Read the model definition and answer for the solid it produces. Units are mm, in the model's axes. A direction names the side the tool comes from. Coordinates: 2 decimals unless noted, no trailing zeros. Loops run counter-clockwise (first coordinate to the right, second up) from the corner with the lowest first, then second, coordinate; pieces in that order, holes last. Notation, with made-up numbers: (26, -5) - (82, -5) arc R23 ccw to (82, 25) - close; hole circle Ø6 at (67.5, 66.25). An arc over 180 degrees is marked (long way). One line per question, with ' | ' between items. Start each with the question number.
```python
from build123d import *

# Parameters (mm, degrees)
F0_W     = 42.25
F0_H     = 214
F1_DEPTH = 59
F3_DEPTH = 214
F4_T     = -1.5


with BuildPart() as f1:
    # F0 (on Top) → F1 (new body)
    with BuildSketch(Plane.XY):
        with Locations((21.125, 107)):
            Rectangle(F0_W, F0_H)
    extrude(amount=F1_DEPTH)

    # F2 (on face) → F3 (cut, through all)
    with BuildSketch(Plane(origin=(0, 214, 0), x_dir=(-1, 0, 0), z_dir=(0, 1, 0))):
        Polygon((0, 0), (-42.25, 59), (-42.25, 0), align=None)
    extrude(amount=-F3_DEPTH, mode=Mode.SUBTRACT)

    # F4
    f4_openings = [f1.faces().sort_by_distance(p)[0] for p in [
        (21.125, 107, 29.5),
    ]]
    offset(amount=F4_T, openings=f4_openings)


solid = f1.part
```
1) Given pin 1 Ø2 at (x, y) = (23.5, 86.5) entering from -Z, flat-ended and moving along its own axis, determine where the tip first touches the part or whether it passes through.
2) Find the intervals of material crossed by line 1 along Y through (x, z) = (23, 42); line 2 along X through (y, z) = (43, 35); line 3 along Z through (x, y) = (18, 165.5), in increasing order. Write a range as from..to.
3) The part is cut by section A-A on y = 92. Write down the section's boundary in (x, z), and give its area (3 significant figures).
4) The part is cut by section C-C on x = 39. Write down the section's boundary in (y, z), and give its area (3 significant figures).
5) The part is cut by section B-B on z = 46. Write down the section's boundary in (x, y), and give its area (3 significant figures).
6) Which of the six approach directions +Z, -Z, +X, -X, +Y, -Y give full straight-line access (tool end or side, diameter ignored) to faces 4 (the flat face through (0, 106, 29)), 5 (the flat face through (1.5, 106, 29))?
7) The mould has two halves that part along Y. Classify faces 1 (the flat face through (21, 108, 59)), 2 (the flat face through (12, 1.5, 42)), 3 (the flat face through (11, 0, 42)): released by +Y, released by -Y, zero draft, split by the parting line, or undercut.
Answer below:
1) pin 1: z = 57.5
2) line 1: 0..1.5, 212.5..214 | line 2: 0..1.5 | line 3: 57.5..59
3) outline: (0, 0) - (1.5, 2.09) - (1.5, 57.5) - (41.18, 57.5) - (42.25, 59) - (0, 59) - close | area: 147 mm2
4) outline: (0, 54.46) - (1.5, 54.46) - (1.5, 57.5) - (212.5, 57.5) - (212.5, 54.46) - (214, 54.46) - (214, 59) - (0, 59) - close | area: 330 mm2
5) outline: (0, 0) - (32.94, 0) - (32.94, 1.5) - (1.5, 1.5) - (1.5, 212.5) - (32.94, 212.5) - (32.94, 214) - (0, 214) - close | area: 415 mm2
6) face 4: +Z, -Z, -X, +Y, -Y | face 5: -Z, +X
7) face 1: zero draft | face 2: undercut | face 3: released by -Y
